```python
from build123d import *

# Parameters (mm, degrees)
F2_R     = 7.5
F4_DEPTH = 33


# Not quite as in the source:
# - a feature of the source that left no trace in its solid (it failed there, or was rolled back) is left out


with BuildPart() as f1:
    # F0 (on Right) → F1 (revolve)
    with BuildSketch(Plane.YZ):
        with BuildLine():
            Line((-13.5163067589, 39), (-21.5163067589, 39))
            Line((-21.5163067589, 39), (-21.5163067589, 32))
            Line((-21.5163067589, 32), (8.4836932411, 29))
            Line((8.4836932411, 29), (8.4836932411, 25))
            Line((8.4836932411, 25), (50.4836932411, 25))
            Line((50.4836932411, 25), (50.4836932411, 0))
            Line((50.4836932411, 0), (68.4836932411, 0))
            Line((68.4836932411, 0), (68.4836932411, 32))
            Line((68.4836932411, 32), (71.4836932411, 32))
            Line((71.4836932411, 32), (71.4836932411, 39))
            Line((71.4836932411, 39), (38.7984625995, 39))
            Line((38.7984625995, 39), (24.3515754229, 28.8841806952))
            ThreePointArc((24.3515754229, 28.8841806952), (19.1749501749, 28.5448867508), (16.4836932411, 32.9799409167))
            Line((16.4836932411, 32.9799409167), (16.4836932411, 45))
            Line((16.4836932411, 45), (-13.5163067589, 45))
            Line((-13.5163067589, 45), (-13.5163067589, 39))
        make_face()
    revolve(axis=Axis((0, 59.4836932411, 0), (0, -1, 0)))

    # F2 (on face) → F4 (join)
    with BuildSketch(Plane(origin=(0, 71.4836932411, 0), x_dir=(-1, 0, 0), z_dir=(0, 1, 0))):
        with BuildLine():
            ThreePointArc((36.6079755837, -13.4482758621), (0, -39), (-36.6079755837, -13.4482758621))
            Line((-36.6079755837, -13.4482758621), (-17.8346547716, -64.5517241379))
            ThreePointArc((-17.8346547716, -64.5517241379), (0, -77), (17.8346547716, -64.5517241379))
            Line((17.8346547716, -64.5517241379), (36.6079755837, -13.4482758621))
        make_face()
        with Locations((0, -58)):
            Circle(F2_R, mode=Mode.SUBTRACT)
        with BuildLine():
            ThreePointArc((17.8346547716, 64.5517241379), (0, 77), (-17.8346547716, 64.5517241379))
            Line((-17.8346547716, 64.5517241379), (-36.6079755837, 13.4482758621))
            ThreePointArc((-36.6079755837, 13.4482758621), (0, 39), (36.6079755837, 13.4482758621))
            Line((36.6079755837, 13.4482758621), (17.8346547716, 64.5517241379))
        make_face()
        with Locations((0, 58)):
            Circle(F2_R, mode=Mode.SUBTRACT)
    extrude(amount=-F4_DEPTH)


solid = f1.part
```
Could you check a few things on this model? Use its own coordinates, in mm. A direction names the side the tool comes from. Coordinates: 2 decimals unless noted, no trailing zeros. Write each loop counter-clockwise with the first axis right and the second up, starting at its lowest first coordinate (ties: lowest second). Pieces come first, ordered by that corner, then holes. Notation, with made-up numbers: (10.5, 42) -> (21.5, 42) arc R26 cw to (21.5, 68) -> close; hole circle Ø2 at (-6, 22). An arc over 180 degrees is marked (long way). Return JSON: item names as keys, results as strings.
(1) We'd pull the mould along Z, two halves only. Please class faces 1 (the cylindrical face through (0, 55, 77)), 2 (the flat face through (-22, 8.484, 13)), 3 (the flat face through (-32, -21.516, 6)), 4 (the flat face through (0, 50.484, 0)): +Z half, -Z half, draft (parallel to the pull), parting line (faces both ways), or undercut.
Numbers:
{"face 1": "+Z half", "face 2": "undercut", "face 3": "draft", "face 4": "undercut"}
(2) Which directions (+Z, -Z, +X, -X, +Y, -Y) give clear straight access to the entire face, cutting with the end or side of a thin tool? Please do faces 5 (the flat face through (-27.353, 55.215, 38.642)), 6 (the cylindrical face through (39, 55, 0)), 7 (the conical face through (28.677, 25.053, -6.368)), 8 (the flat face through (1, 38.484, 46)), 9 (the cylindrical face through (-7.509, 29.778, 23.846)).
Numbers:
{"face 5": "+Z, -X, +Y", "face 6": "+X, +Y", "face 7": "none", "face 8": "+Z", "face 9": "-Y"}
(3) I need wall thicknesses on L1, parallel to Y at x = 25, z = 30.5; L2, parallel to Y at x = 1.5, z = -24; L3, parallel to Z at x = 5.5, y = -15.5. Which ranges of each line are inside material? Lowest first, please.
Numbers:
{"L1": "y = -13.52 to 16.48, 38.48 to 71.48", "L2": "y = 50.48 to 68.48", "L3": "z = -38.61 to -30.91, 30.91 to 38.61"}
(4) Imagine slicing it at D-D, the plane z = 0. Please give me the cut outline in (x, y).
Numbers:
{"outline": "(-45, -13.52) -> (-39, -13.52) -> (-39, -21.52) -> (-32, -21.52) -> (-29, 8.48) -> (-25, 8.48) -> (-25, 50.48) -> (25, 50.48) -> (25, 8.48) -> (29, 8.48) -> (32, -21.52) -> (39, -21.52) -> (39, -13.52) -> (45, -13.52) -> (45, 16.48) -> (32.98, 16.48) arc R5 cw to (28.88, 24.35) -> (39, 38.8) -> (39, 71.48) -> (32, 71.48) -> (32, 68.48) -> (-32, 68.48) -> (-32, 71.48) -> (-39, 71.48) -> (-39, 38.8) -> (-28.88, 24.35) arc R5 cw to (-32.98, 16.48) -> (-45, 16.48) -> close"}
(5) I'm going to push flat-ended pins straight in: pin 1 (4 mm diameter, centred on x = -5, y = 15.5, fed in from +Z); pin 2 (8 mm diameter, centred on x = 5.5, y = 23, fed in from +Z); pin 3 (2 mm diameter, centred on y = 35, z = -16.5, fed in from -X). Where does each tip first touch, or does it pass through?
Numbers:
{"pin 1": "stops at z = 44.9", "pin 2": "stops at z = 30.32", "pin 3": "stops at x = -33.3"}
(6) Imagine slicing it at A-A, the plane y = 57.5. Please give me the cut outline in (x, z).
Numbers:
{"outline": "(-36.61, -13.45) -> (-17.83, -64.55) arc R19 ccw to (17.83, -64.55) -> (36.61, -13.45) arc R39 ccw to (36.61, 13.45) -> (17.83, 64.55) arc R19 ccw to (-17.83, 64.55) -> (-36.61, 13.45) arc R39 ccw to start; hole circle Ø15 at (0, -58); hole circle Ø15 at (0, 58)"}
(7) Imagine slicing it at C-C, the plane y = 14. Please give me the cut outline in (x, z).
Numbers:
{"outline": "circle Ø90 at (0, 0); hole circle Ø50 at (0, 0)"}
(8) Imagine slicing it at B-B, the plane z = -58. Please give me the cut outline in (x, y), then the cut area to 3 significant figures.
Numbers:
{"outline": "(-20.24, 38.48) -> (-7.5, 38.48) -> (-7.5, 71.48) -> (-20.24, 71.48) -> close; (7.5, 38.48) -> (20.24, 38.48) -> (20.24, 71.48) -> (7.5, 71.48) -> close", "area": "841 mm2"}
